```python
from build123d import *

# Parameters (mm, degrees)
BOSS_EXTRUDE1_DEPTH = 10
SKETCH2_R           = 16.25
BOSS_EXTRUDE2_DEPTH = 10
SKETCH3_R           = 5
CUT_EXTRUDE1_DEPTH  = 10


with BuildPart() as part:
    # Sketch1 → Boss-Extrude1 (new body)
    with BuildSketch(Plane(origin=(0, 0, 0), x_dir=(1, 0, 0), z_dir=(0, 0, -1))):
        with BuildLine():
            Line((18.95720217, -67.165147363), (67.645318019, 17.165182331))
            ThreePointArc((67.645318019, 17.165182331), (74.442164244, 23.570200009), (83.642337861, 25.175869802))
            ThreePointArc((83.642337861, 25.175869802), (108.253132571, 62.500004371), (63.624087575, 59.848480209))
            ThreePointArc((63.624087575, 59.848480209), (57.63345283, 52.683728615), (48.68812278, 49.999992345))
            Line((48.68812278, 49.999992345), (-48.688142969, 49.999972686))
            ThreePointArc((-48.688142969, 49.999972686), (-57.633474102, 52.683705343), (-63.624111741, 59.848454519))
            ThreePointArc((-63.624111741, 59.848454519), (-108.253157807, 62.49996066), (-83.642348027, 25.175836028))
            ThreePointArc((-83.642348027, 25.175836028), (-74.442173761, 23.570169951), (-67.64532495, 17.165155017))
            Line((-67.64532495, 17.165155017), (-18.95717505, -67.165155017))
            ThreePointArc((-18.95717505, -67.165155017), (-16.808690142, -76.253905353), (-20.01822612, -85.02432432))
            ThreePointArc((-20.01822612, -85.02432432), (2.5237e-05, -124.999965031), (20.018260452, -85.024316237))
            ThreePointArc((20.018260452, -85.024316237), (16.808720932, -76.253898566), (18.95720217, -67.165147363))
        make_face()
    extrude(amount=BOSS_EXTRUDE1_DEPTH)

    # Sketch2 → Boss-Extrude2 (add)
    with BuildSketch(Plane(origin=(0, 0, -10), x_dir=(1, 0, 0), z_dir=(0, 0, -1))):
        with Locations((86.6025, 50)):
            Circle(SKETCH2_R)
        with Locations((2.0189e-05, -99.999965031)):
            Circle(SKETCH2_R)
        with Locations((-86.602520189, 49.999965031)):
            Circle(SKETCH2_R)
    extrude(amount=BOSS_EXTRUDE2_DEPTH)

    # Sketch3 → Cut-Extrude1 (cut)
    with BuildSketch(Plane.XY):
        Circle(SKETCH3_R)
    extrude(amount=-CUT_EXTRUDE1_DEPTH, mode=Mode.SUBTRACT)


solid = part.part
```
Geometry check sheet. Reference: the model listing, model coordinates, mm. A direction names the side the tool comes from. Coordinates: 2 decimals unless noted, no trailing zeros. Write each loop counter-clockwise with the first axis right and the second up, starting at its lowest first coordinate (ties: lowest second). Pieces come first, ordered by that corner, then holes. Notation, with made-up numbers: M 37,10 L 52,10 A12 ccw 52,18 Z; hole C -37.75,-16 d10. An arc over 180 degrees is marked long. One line per item, written item: value. Start each with the question number.
(1) Depth check by flat-ended pin: pin 1 (10 mm diameter, centred on x = 20, z = -17.5, fed in from -Y); pin 2 (5 mm diameter, centred on x = 52.5, y = 3, fed in from -Z); pin 3 (3 mm diameter, centred on x = 13.5, z = -7.5, fed in from -Y). Enter the tip coordinate at first touch or a pass-through.
(2) Sectioned sample at D-D, the plane x = -95. Enter the section's corners in (y, z), and give its area (3 significant figures).
(3) Sectioned sample at B-B, the plane y = 0. Enter the section's corners in (x, z) (3 decimals).
(4) Scan lines: line 1 along Y through (x, z) = (0, -3); line 2 along Z through (x, y) = (-65.5, -28); line 3 along X through (y, z) = (61, -3.5). Record each from-to range of solid material in increasing order. Write a range as [from, to].
(5) Release check for a two-part mould opening along X. For faces 1 (the face through (74.3, -23.5, -4.9)), 2 (the face through (-57.52, -52.61, -4.93)), 3 (the face through (16.817, 76.386, -4.93)), 4 (the face through (-2.12, 83.89, -14.93)) record: released by +X, released by -X, zero draft, split by the parting line, or undercut.
(6) Sectioned sample at A-A, the plane x = 0. Enter the section's corners in (y, z).
(7) Sectioned sample at C-C, the plane z = -7. Enter the section's corners in (x, y).
(8) Tool access check on faces 5 (the face through (-98.58, -60.98, -14.93)), 6 (the face through (1, -50, -5)), 7 (the face through (-74.56, -23.63, -4.93)). Record the directions out of +Z, -Z, +X, -X, +Y, -Y that give a thin tool (end or side, any length) a straight path to the whole face; none if there is none.
Filled sheet:
1. pin 1: y = 93.75
1. pin 2: z = -10
1. pin 3: y = -50
2. outline: M -73.55,-10 L -63.91,-10 L -63.91,-20 L -36.09,-20 L -36.09,-10 L -26.45,-10 L -26.45,0 L -73.55,0 Z
2. area: 749 mm²
3. outline: M -57.735,-10 L -5,-10 L -5,0 L -57.735,0 Z; M 5,-10 L 57.735,-10 L 57.735,0 L 5,0 Z
4. line 1: [-50, -5], [5, 125]
4. line 2: [-10, 0]
4. line 3: [-22.52, 22.52]
5. face 1: undercut
5. face 2: undercut
5. face 3: released by +X
5. face 4: split by the parting line
6. outline: M -50,-10 L -5,-10 L -5,0 L -50,0 Z; M 5,-10 L 83.75,-10 L 83.75,-20 L 116.25,-20 L 116.25,-10 L 125,-10 L 125,0 L 5,0 Z
7. outline: M -83.64,-25.18 A25 ccw long -63.62,-59.85 A16.25 cw -48.69,-50 L 48.69,-50 A16.25 cw 63.62,-59.85 A25 ccw long 83.64,-25.18 A16.25 cw 67.65,-17.17 L 18.96,67.17 A16.25 cw 20.02,85.02 A25 ccw long -20.02,85.02 A16.25 cw -18.96,67.17 L -67.65,-17.17 A16.25 cw Z; hole C 0,0 d10
8. face 5: -Z
8. face 6: +Z, -Z, -Y
8. face 7: +Z, -Z, +Y
